Input: part model. Units: mm. Frame: model coordinates. Give positions to 0.01 mm unless a question says otherwise; leave off trailing zeros. Loops run counter-clockwise (first coordinate to the right, second up) from the corner with the lowest first, then second, coordinate; pieces in that order, holes last.
from build123d import *

# Parameters (mm, degrees)
SKETCH_3_W      = 40
SKETCH_3_H      = 15
EXTRUDE_2_DEPTH = 3
FILLET1_R       = 15


with BuildPart() as part:
    # Эскиз3 → Бобышка-Вытянуть2 (new body)
    with BuildSketch(Plane(origin=(0, 0, 0), x_dir=(1, 0, 0), z_dir=(0, 1, 0))):
        Polygon((0, 52), (3, 52), (3, 58), (6, 58), (6, 56.5), (40, 56.5), (40, 53.5), (70, 53.5), (70, 56.5), (104, 56.5), (104, 58), (107, 58), (107, 52), (110, 52), (110, 0), (58, 0), (58, 3), (55, 3), (52, 3), (52, 0), (0, 0), align=None)
        with Locations((55, 26)):
            Rectangle(SKETCH_3_W, SKETCH_3_H, mode=Mode.SUBTRACT)
    extrude(amount=EXTRUDE_2_DEPTH)

    # Fillet1
    fillet1_edges = [part.edges().sort_by_distance(p)[0] for p in [
        (110, 1.5, 0),
        (0, 1.5, 0),
    ]]
    fillet(fillet1_edges, radius=FILLET1_R)


solid = part.part
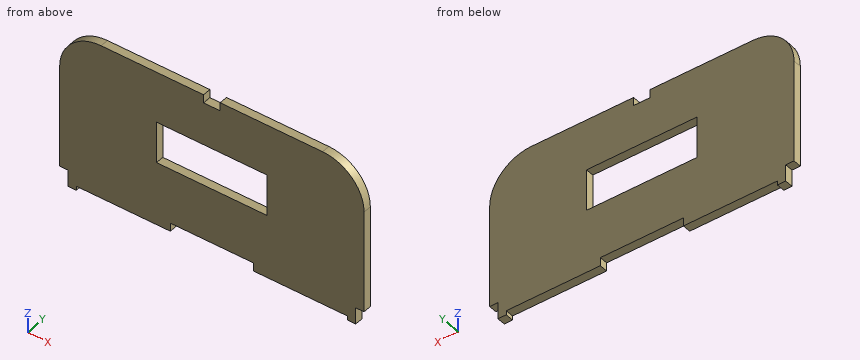
(1) Pin query (flat end, axial travel): pin 1 Ø1.6 at (y, z) = (1.5, -57.5) entering from -X; pin 2 Ø0.9 at (x, y) = (46, 2) entering from -Z; pin 3 Ø0.9 at (y, z) = (2, -1) entering from -X. Return the tip coordinate at first contact, or that it passes through.
Values follow:
pin 1: stops at x = 3
pin 2: stops at z = -53.5
pin 3: stops at x = 8.57
(2) Cut plane A-A (x = 42.5). Return the cut outline in (y, z).
Values follow:
outline: (0, -53.5) - (3, -53.5) - (3, -33.5) - (0, -33.5) - close; (0, -18.5) - (3, -18.5) - (3, 0) - (0, 0) - close
(3) Cut plane D-D (x = 81.5). Return the cut outline in (y, z).
Values follow:
outline: (0, -56.5) - (3, -56.5) - (3, 0) - (0, 0) - close
(4) Cut plane B-B (z = -31.5). Return the cut outline in (x, y), and give its area (3 significant figures).
Values follow:
outline: (0, 0) - (35, 0) - (35, 3) - (0, 3) - close; (75, 0) - (110, 0) - (110, 3) - (75, 3) - close
area: 210 mm2
(5) Cut plane C-C (y = 0.75). Return the cut outline in (x, z).
Values follow:
outline: (0, -52) - (3, -52) - (3, -58) - (6, -58) - (6, -56.5) - (40, -56.5) - (40, -53.5) - (70, -53.5) - (70, -56.5) - (104, -56.5) - (104, -58) - (107, -58) - (107, -52) - (110, -52) - (110, -15) arc R15 ccw to (95, 0) - (58, 0) - (58, -3) - (52, -3) - (52, 0) - (15, 0) arc R15 ccw to (0, -15) - close; hole (35, -33.5) - (75, -33.5) - (75, -18.5) - (35, -18.5) - close
(6) Ray query, probe 1 along Z at (x, y) = (60, 1.9); probe 2 along X at (y, z) = (2.75, -25); probe 3 along X at (y, z) = (1.1, -54.5). Return the intervals inside material, ascending.
Values follow:
probe 1: z = -53.5 to -33.5, -18.5 to 0
probe 2: x = 0 to 35, 75 to 110
probe 3: x = 3 to 40, 70 to 107
